Read the model definition and answer for the solid it produces. Units are mm, in the model's axes. Round coordinates to 2 decimals unless told otherwise and drop trailing zeros. Order: outer loops, then holes, each group sorted by start corner. A loop starts at its lowest first (then second) coordinate and runs counter-clockwise, first axis right, second up. Notation, with made-up numbers: (-33, 21) - (-22, 21) arc R18 cw to (-22, 41) - close; hole circle Ø1 at (81, 39.25). An arc over 180 degrees is marked (long way). Answer as a JSON object with one key per item and string values. Group by question number.
Q1. Given pin 1 Ø10 at (y, z) = (-27.5, 19.5) entering from +X; pin 2 Ø2 at (x, y) = (10, -26) entering from +Z; pin 3 Ø4 at (x, z) = (-14, 0) entering from -Y; pin 4 Ø10 at (y, z) = (-11.5, -54.5) entering from +X, each flat-ended and moving along its own axis, determine where each tip first touches the part or whether it passes through.
Q2. A cutting plane is placed at C-C on z = 35. Determine the outline of the cut face in (x, y) (3 decimals).
Q3. The mould has two halves that part along Z. Classify faces 1 (the flat face through (-31.737, -7.605, 24.063)), 2 (the cylindrical face through (21.78, -19.72, 69.15)): pulls with the +Z half, pulls with the -Z half, needs draft (parallel to the pull), parting line crosses it, or undercut.
Q4. A cutting plane is placed at B-B on z = 14. Determine the outline of the cut face in (x, y), and give its area (3 significant figures).
Q5. A cutting plane is placed at A-A on x = 0. Determine the outline of the cut face in (y, z).
Q6. Consider line 1 (Z direction, x = 25.5, y = -4.5); line 2 (Z direction, x = -37.5, y = -7); line 3 (X direction, y = -3.5, z = -20.5). Determine where each line is inside the solid, lowest interval first.
Q7. A cutting plane is placed at D-D on y = -19.5. Determine the outline of the cut face in (x, z).
```python
from build123d import *

# Parameters (mm, degrees)
SKETCH1_R           = 72.5
SKETCH1_R_2         = 64.5
BOSS_EXTRUDE1_DEPTH = 40
SKETCH4_R           = 64.5
BOSS_EXTRUDE3_DEPTH = 15
SKETCH3_R           = 2.5
CUT_EXTRUDE1_DEPTH  = 15
SKETCH6_R           = 2.5
CUT_EXTRUDE2_DEPTH  = 30
SKETCH7_R           = 72.5
CUT_EXTRUDE3_DEPTH  = 40


with BuildPart() as part:
    # Sketch1 → Boss-Extrude1 (new, symmetric)
    with BuildSketch(Plane(origin=(0, 0, 0), x_dir=(1, 0, 0), z_dir=(0, 1, 0))):
        with Locations(Location((0, 0, 0), (0, 0, 270))):
            Circle(SKETCH1_R)
        with Locations(Location((0, 0, 0), (0, 0, 270))):
            Circle(SKETCH1_R_2, mode=Mode.SUBTRACT)
    extrude(amount=BOSS_EXTRUDE1_DEPTH, both=True)

    # Sketch4 → Boss-Extrude3 (add, symmetric)
    with BuildSketch(Plane(origin=(0, 0, 0), x_dir=(1, 0, 0), z_dir=(0, 1, 0))):
        with Locations(Location((0, 0, 0), (0, 0, 270))):
            Circle(SKETCH4_R)
    extrude(amount=BOSS_EXTRUDE3_DEPTH, both=True)

    # Sketch3 → Cut-Extrude1 (cut, symmetric)
    with BuildSketch(Plane.XZ):
        with Locations(Location((-34.091544633, 46.922985674, 0), (0, 0, 270))):
            Circle(SKETCH3_R)
        with Locations(Location((34.091544633, 46.922985674, 0), (0, 0, 270))):
            Circle(SKETCH3_R)
        with Locations(Location((55.161277945, -17.922985674, 0), (0, 0, 270))):
            Circle(SKETCH3_R)
        with Locations(Location((0, -58, 0), (0, 0, 270))):
            Circle(SKETCH3_R)
        with Locations(Location((-55.161277945, -17.922985674, 0), (0, 0, 270))):
            Circle(SKETCH3_R)
        with BuildLine():
            Line((8.942342186, 26.255693464), (17.100089792, 48.668920804))
            ThreePointArc((17.100089792, 48.668920804), (16.728172015, 53.596235201), (12.784464921, 56.573469548))
            ThreePointArc((12.784464921, 56.573469548), (0, 58), (-12.784464921, 56.573469548))
            ThreePointArc((-12.784464921, 56.573469548), (-16.728172015, 53.596235201), (-17.100089792, 48.668920804))
            Line((-17.100089792, 48.668920804), (-8.942342186, 26.255693464))
            ThreePointArc((-8.942342186, 26.255693464), (-6.454448371, 23.201362532), (-2.608568259, 22.348274467))
            ThreePointArc((-2.608568259, 22.348274467), (0, 22.5), (2.608568259, 22.348274467))
            ThreePointArc((2.608568259, 22.348274467), (6.454448371, 23.201362532), (8.942342186, 26.255693464))
        make_face()
        with BuildLine():
            Line((22.207312654, 16.618128287), (41.002675921, 31.302675452))
            ThreePointArc((41.002675921, 31.302675452), (45.803759299, 32.471584512), (49.853949939, 29.640912191))
            ThreePointArc((49.853949939, 29.640912191), (55.525129356, 16.76186177), (57.927651105, 2.896072756))
            ThreePointArc((57.927651105, 2.896072756), (56.782266496, -0.110724751), (53.793042698, -1.301219707))
            Line((53.793042698, -1.301219707), (27.733984064, -0.391217328))
            ThreePointArc((27.733984064, -0.391217328), (24.060341259, 1.031070133), (22.060563983, 4.425100764))
            ThreePointArc((22.060563983, 4.425100764), (21.398771617, 6.952882373), (20.448380136, 9.386892446))
            ThreePointArc((20.448380136, 9.386892446), (20.071272788, 13.308160497), (22.207312654, 16.618128287))
        make_face()
        with BuildLine():
            Line((22.667216205, -15.985125354), (42.44113714, -29.322803436))
            ThreePointArc((42.44113714, -29.322803436), (45.036452074, -33.527692304), (43.595900456, -38.254378356))
            ThreePointArc((43.595900456, -38.254378356), (34.091544633, -46.922985674), (22.910201686, -53.283418234))
            ThreePointArc((22.910201686, -53.283418234), (17.969701185, -53.19283792), (14.772610647, -49.42516462))
            Line((14.772610647, -49.42516462), (8.198202609, -26.49747907))
            ThreePointArc((8.198202609, -26.49747907), (8.415660309, -22.564126145), (11.025610093, -19.613411791))
            ThreePointArc((11.025610093, -19.613411791), (13.225168177, -18.202882373), (15.246362198, -16.546855886))
            ThreePointArc((15.246362198, -16.546855886), (18.859177151, -14.976467017), (22.667216205, -15.985125354))
        make_face()
        with BuildLine():
            Line((-8.198202609, -26.49747907), (-14.772610647, -49.42516462))
            ThreePointArc((-14.772610647, -49.42516462), (-17.969701185, -53.19283792), (-22.910201686, -53.283418234))
            ThreePointArc((-22.910201686, -53.283418234), (-34.091544633, -46.922985674), (-43.595900456, -38.254378356))
            ThreePointArc((-43.595900456, -38.254378356), (-45.036452074, -33.527692304), (-42.44113714, -29.322803436))
            Line((-42.44113714, -29.322803436), (-22.667216205, -15.985125354))
            ThreePointArc((-22.667216205, -15.985125354), (-18.859177151, -14.976467017), (-15.246362198, -16.546855886))
            ThreePointArc((-15.246362198, -16.546855886), (-13.225168177, -18.202882373), (-11.025610093, -19.613411791))
            ThreePointArc((-11.025610093, -19.613411791), (-8.415660309, -22.564126145), (-8.198202609, -26.49747907))
        make_face()
        with BuildLine():
            Line((-27.733984064, -0.391217328), (-51.571112622, -1.223628199))
            ThreePointArc((-51.571112622, -1.223628199), (-56.142338174, 0.652710511), (-57.755183787, 5.323414851))
            ThreePointArc((-57.755183787, 5.323414851), (-55.161277945, 17.922985674), (-49.853949939, 29.640912191))
            ThreePointArc((-49.853949939, 29.640912191), (-45.803759299, 32.471584512), (-41.002675921, 31.302675452))
            Line((-41.002675921, 31.302675452), (-22.207312654, 16.618128287))
            ThreePointArc((-22.207312654, 16.618128287), (-20.071272788, 13.308160497), (-20.448380136, 9.386892446))
            ThreePointArc((-20.448380136, 9.386892446), (-21.398771617, 6.952882373), (-22.060563983, 4.425100764))
            ThreePointArc((-22.060563983, 4.425100764), (-24.060341259, 1.031070133), (-27.733984064, -0.391217328))
        make_face()
    extrude(amount=CUT_EXTRUDE1_DEPTH, both=True, mode=Mode.SUBTRACT)

    # Sketch6 → Cut-Extrude2 (cut)
    with BuildSketch(Plane(origin=(0, 15, 0), x_dir=(1, 0, 0), z_dir=(0, 1, 0))):
        with Locations(Location((0, 14, 0), (0, 0, 270))):
            Circle(SKETCH6_R)
        with Locations(Location((14, 0, 0), (0, 0, 270))):
            Circle(SKETCH6_R)
        with Locations(Location((0, -14, 0), (0, 0, 270))):
            Circle(SKETCH6_R)
        with Locations(Location((-14, 0, 0), (0, 0, 270))):
            Circle(SKETCH6_R)
    extrude(amount=-CUT_EXTRUDE2_DEPTH, mode=Mode.SUBTRACT)

    # Sketch7 → Cut-Extrude3 (cut)
    with BuildSketch(Plane(origin=(0, 40, 0), x_dir=(1, 0, 0), z_dir=(0, 1, 0))):
        with Locations(Location((0, 0, 0), (0, 0, 270))):
            Circle(SKETCH7_R)
    extrude(amount=-CUT_EXTRUDE3_DEPTH, mode=Mode.SUBTRACT)


solid = part.part
```
Result set:
{
 "1": {"pin 1": "stops at x = 71.04", "pin 2": "stops at z = 71.94", "pin 3": "passes through", "pin 4": "stops at x = 52.97"},
 "2": {"outline": "(-63.492, -40) - (-54.178, -40) - (-54.178, -15) - (-12.125, -15) - (-12.125, 0) - (-63.492, 0) - close; (12.125, -15) - (54.178, -15) - (54.178, -40) - (63.492, -40) - (63.492, 0) - (12.125, 0) - close"},
 "3": {"face 1": "undercut", "face 2": "parting line crosses it"},
 "4": {"outline": "(-71.14, -40) - (-62.96, -40) - (-62.96, -15) - (-56.28, -15) - (-56.28, 0) - (-71.14, 0) - close; (-20.28, -15) - (-2.5, -15) - (-2.5, 0) - (-20.28, 0) - close; (2.5, -15) - (20.28, -15) - (20.28, 0) - (2.5, 0) - close; (56.28, -15) - (62.96, -15) - (62.96, -40) - (71.14, -40) - (71.14, 0) - (56.28, 0) - close", "area": "1,390 mm²"},
 "5": {"outline": "(-40, -72.5) - (0, -72.5) - (0, -60.5) - (-15, -60.5) - (-15, -64.5) - (-40, -64.5) - close; (-40, 64.5) - (-15, 64.5) - (-15, 58) - (0, 58) - (0, 72.5) - (-40, 72.5) - close; (-15, -55.5) - (0, -55.5) - (0, -16.5) - (-15, -16.5) - close; (-15, -11.5) - (0, -11.5) - (0, 11.5) - (-15, 11.5) - close; (-15, 16.5) - (0, 16.5) - (0, 22.5) - (-15, 22.5) - close"},
 "6": {"line 1": "z = -67.87 to -52.09, -17.9 to 0.13, 19.19 to 67.87", "line 2": "z = -62.05 to -44.25, -25.99 to -0.73, 28.57 to 62.05", "line 3": "x = -69.54 to -29.36, -9.83 to 9.83, 29.36 to 69.54"},
 "7": {"outline": "circle Ø145 at (0, 0); hole circle Ø129 at (0, 0)"}
}
